Input: part model. Units: mm. Frame: model coordinates. A direction names the side the tool comes from. Round coordinates to 2 decimals unless told otherwise and drop trailing zeros. Loops run counter-clockwise (first coordinate to the right, second up) from the corner with the lowest first, then second, coordinate; pieces in that order, holes last. Notation, with made-up numbers: (-21.75, 20.25) -> (-12.75, 20.25) arc R22 ccw to (-12.75, 59.25) -> close; hole circle Ø5 at (19, 33.5). An arc over 180 degrees is marked (long way). One line per question, with ' | ' between items. Start each with the question number.
Q1. Cut plane B-B on z = -56. State how many separate pieces and enclosed holes the cut face has, and give its area (3 significant figures).
Q2. Access query for faces 1 (the face through (338, -104, 10)), 2 (the face through (310, -101, -1)), 3 (the face through (10, -94, 59)). Directions: +Z, -Z, +X, -X, +Y, -Y. A direction counts if a zero-diameter tool reaches every point of the face in a straight line with its end or side. Return the directions, or none.
Q3. Cut plane A-A on x = 233.5. Return loops of the section in (y, z).
Q4. Material intervals for L1, parallel to Y at x = 18.5, z = 80.5; L2, parallel to X at y = -103.5, z = 90; L3, parallel to X at y = 5, z = -18, sorted ascending.
Q5. Mould query, pull axis X, two halves, no side actions, for faces 4 (the face through (307.15, -101.4, 101.99)), 5 (the face through (205, 114, 116)). Classes: pulls with the +X half, pulls with the -X half, needs draft (parallel to the pull), parting line crosses it, or undercut.
Q6. Contact query for flat-ended pins moving along their axis: P1, Ø4, axis at y = -29, z = 47.5, coming from the -X side; P2, Ø8, axis at x = 191, y = -87.5, coming from the +Z side; P3, Ø10, axis at y = -101.5, z = 44, coming from the -X side; P4, Ø4, axis at x = 328, z = -9.5, coming from the +Y side. Output: stop coordinate, or through.
Q7. Cut plane D-D on y = 65.5. Return loops of the section in (x, z), and give its area (3 significant figures).
Q8. Cut plane C-C on x = 38. Return loops of the section in (y, z).
from build123d import *

# Parameters (mm, degrees)
SKETCH1_W            = 20
SKETCH1_H            = 260
BOSS_EXTRUDE1_DEPTH  = 10
CUT_EXTRUDE1_DEPTH   = 15
SKETCH3_W            = 10
SKETCH3_H            = 20
BOSS_EXTRUDE2_DEPTH  = 40
BOSS_EXTRUDE3_DEPTH  = 230
BOSS_EXTRUDE4_DEPTH  = 50
SKETCH6_W            = 260
SKETCH6_H            = 228
BOSS_EXTRUDE5_DEPTH  = 20
SKETCH7_W            = 20
SKETCH7_H            = 17
BOSS_EXTRUDE6_DEPTH  = 50
SKETCH8_W            = 20
SKETCH8_H            = 60
BOSS_EXTRUDE7_DEPTH  = 50
SKETCH9_W            = 20
SKETCH9_H            = 60
BOSS_EXTRUDE8_DEPTH  = 50
SKETCH10_W           = 20
SKETCH10_H           = 20
BOSS_EXTRUDE9_DEPTH  = 340
SKETCH11_W           = 20
SKETCH11_H           = 20
BOSS_EXTRUDE10_DEPTH = 340
SKETCH12_W           = 260
SKETCH12_H           = 228
BOSS_EXTRUDE11_DEPTH = 20
SKETCH13_W           = 40
SKETCH13_H           = 20
CUT_EXTRUDE2_DEPTH   = 240
SKETCH14_W           = 210
SKETCH14_H           = 15
CUT_EXTRUDE3_DEPTH   = 230
SKETCH15_W           = 100
SKETCH15_H           = 20
CUT_EXTRUDE4_DEPTH   = 45
SKETCH16_W           = 20
SKETCH16_H           = 100
CUT_EXTRUDE5_DEPTH   = 84
SKETCH17_W           = 20
SKETCH17_H           = 100
CUT_EXTRUDE6_DEPTH   = 84
SKETCH18_W           = 20
SKETCH18_H           = 84
CUT_EXTRUDE7_DEPTH   = 100
SKETCH19_W           = 100
SKETCH19_H           = 20
CUT_EXTRUDE8_DEPTH   = 45
CUT_EXTRUDE9_REACH   = 475.244
SKETCH20_W           = 50
SKETCH20_H           = 40
SKETCH21_W           = 50
SKETCH21_H           = 40
CUT_EXTRUDE10_DEPTH  = 18
CUT_EXTRUDE11_REACH  = 475.244
SKETCH22_W           = 50
SKETCH22_H           = 40
SKETCH23_W           = 50
SKETCH23_H           = 40
CUT_EXTRUDE12_DEPTH  = 18
CUT_EXTRUDE13_DEPTH  = 400.369503092
CUT_EXTRUDE14_DEPTH  = 400.369503092
CUT_EXTRUDE15_REACH  = 419.488
FILLET1_R            = 10


with BuildPart() as part:
    # Sketch1 → Boss-Extrude1 (new body)
    with BuildSketch(Plane(origin=(70, 0, 0), x_dir=(0, -1, 0), z_dir=(-1, 0, 0))):
        with Locations((104, 0)):
            Rectangle(SKETCH1_W, SKETCH1_H)
    extrude(amount=-BOSS_EXTRUDE1_DEPTH)

    # Sketch2 → Cut-Extrude1 (cut)
    with BuildSketch(Plane(origin=(0, -94, 0), x_dir=(-1, 0, 0), z_dir=(0, 1, 0))):
        with BuildLine():
            Line((-80, 105), (-80, -105))
            ThreePointArc((-80, -105), (-72.928932188, -102.071067812), (-70, -95))
            Line((-70, -95), (-70, 95))
            ThreePointArc((-70, 95), (-72.928932188, 102.071067812), (-80, 105))
        make_face()
    extrude(amount=-CUT_EXTRUDE1_DEPTH, mode=Mode.SUBTRACT)

    # Sketch3 → Boss-Extrude2 (add)
    with BuildSketch(Plane(origin=(0, -94, 0), x_dir=(-1, 0, 0), z_dir=(0, 1, 0))):
        with Locations((-75, -120)):
            Rectangle(SKETCH3_W, SKETCH3_H)
    extrude(amount=BOSS_EXTRUDE2_DEPTH)

    # Sketch4 → Boss-Extrude3 (add)
    with BuildSketch(Plane(origin=(80, 0, 0), x_dir=(0, 0, -1), z_dir=(1, 0, 0))):
        Polygon((-130, -114), (-130, -94), (110, -94), (110, -54), (130, -54), (130, -114), align=None)
    extrude(amount=BOSS_EXTRUDE3_DEPTH)

    # Sketch5 → Boss-Extrude4 (add)
    with BuildSketch(Plane(origin=(310, 0, 0), x_dir=(0, 0, -1), z_dir=(1, 0, 0))):
        Polygon((110, -94), (110, -54), (130, -54), (130, -114), (-130, -114), (-130, -54), (-110, -54), (-110, -94), align=None)
    extrude(amount=BOSS_EXTRUDE4_DEPTH)

    # Sketch6 → Boss-Extrude5 (add)
    with BuildSketch(Plane(origin=(360, 0, 0), x_dir=(0, 0, -1), z_dir=(1, 0, 0))):
        Rectangle(SKETCH6_W, SKETCH6_H)
        Polygon((92.025912459, -94), (0, -13.30035369), (-92.025912459, -94), align=None, mode=Mode.SUBTRACT)
    extrude(amount=BOSS_EXTRUDE5_DEPTH)

    # Sketch7 → Boss-Extrude6 (add)
    with BuildSketch(Plane.ZY.offset(-70)):
        with Locations((0, -105.5)):
            Rectangle(SKETCH7_W, SKETCH7_H)
    extrude(amount=BOSS_EXTRUDE6_DEPTH)

    # Sketch8 → Boss-Extrude7 (add)
    with BuildSketch(Plane.ZY.offset(-70)):
        with Locations((120, -84)):
            Rectangle(SKETCH8_W, SKETCH8_H)
    extrude(amount=BOSS_EXTRUDE7_DEPTH)

    # Sketch9 → Boss-Extrude8 (add)
    with BuildSketch(Plane.ZY.offset(-70)):
        with Locations((-120, -84)):
            Rectangle(SKETCH9_W, SKETCH9_H)
    extrude(amount=BOSS_EXTRUDE8_DEPTH)

    # Sketch10 → Boss-Extrude9 (add)
    with BuildSketch(Plane.ZY.offset(-360)):
        with Locations((-120, 104)):
            Rectangle(SKETCH10_W, SKETCH10_H)
    extrude(amount=BOSS_EXTRUDE9_DEPTH)

    # Sketch11 → Boss-Extrude10 (add)
    with BuildSketch(Plane.ZY.offset(-360)):
        with Locations((120, 104)):
            Rectangle(SKETCH11_W, SKETCH11_H)
    extrude(amount=BOSS_EXTRUDE10_DEPTH)

    # Sketch12 → Boss-Extrude11 (add)
    with BuildSketch(Plane(origin=(20, 0, 0), x_dir=(0, 0, -1), z_dir=(1, 0, 0))):
        Rectangle(SKETCH12_W, SKETCH12_H)
        Polygon((10, 8.769230769), (10, 10), (11.403508772, 10), align=None, mode=Mode.SUBTRACT)
        Polygon((-10, -94), (-110, -94), (-110, -10), (-11.403508772, -10), (-10, -8.769230769), align=None, mode=Mode.SUBTRACT)
    extrude(amount=-BOSS_EXTRUDE11_DEPTH)

    # Sketch13 → Cut-Extrude2 (cut)
    with BuildSketch(Plane(origin=(70, 0, 0), x_dir=(0, -1, 0), z_dir=(-1, 0, 0))):
        with Locations((74, -120)):
            Rectangle(SKETCH13_W, SKETCH13_H)
    extrude(amount=-CUT_EXTRUDE2_DEPTH, mode=Mode.SUBTRACT)

    # Sketch14 → Cut-Extrude3 (cut)
    with BuildSketch(Plane.ZY.offset(-80)):
        with Locations((0, -101.5)):
            Rectangle(SKETCH14_W, SKETCH14_H)
    extrude(amount=-CUT_EXTRUDE3_DEPTH, mode=Mode.SUBTRACT)

    # Sketch15 → Cut-Extrude4 (cut)
    with BuildSketch(Plane(origin=(360, 0, 0), x_dir=(0, 0, -1), z_dir=(1, 0, 0))):
        with Locations((60, -104)):
            Rectangle(SKETCH15_W, SKETCH15_H)
    extrude(amount=-CUT_EXTRUDE4_DEPTH, mode=Mode.SUBTRACT)

    # Sketch16 → Cut-Extrude5 (cut)
    with BuildSketch(Plane.XZ.offset(-10)):
        with Locations((10, 60)):
            Rectangle(SKETCH16_W, SKETCH16_H)
    extrude(amount=-CUT_EXTRUDE5_DEPTH, mode=Mode.SUBTRACT)

    # Sketch17 → Cut-Extrude6 (cut)
    with BuildSketch(Plane.XZ.offset(-10)):
        with Locations((10, -60)):
            Rectangle(SKETCH17_W, SKETCH17_H)
    extrude(amount=-CUT_EXTRUDE6_DEPTH, mode=Mode.SUBTRACT)

    # Sketch18 → Cut-Extrude7 (cut)
    with BuildSketch(Plane(origin=(0, 0, -110), x_dir=(-1, 0, 0), z_dir=(0, 0, -1))):
        with Locations((-10, -52)):
            Rectangle(SKETCH18_W, SKETCH18_H)
    extrude(amount=-CUT_EXTRUDE7_DEPTH, mode=Mode.SUBTRACT)

    # Sketch19 → Cut-Extrude8 (cut)
    with BuildSketch(Plane(origin=(360, 0, 0), x_dir=(0, 0, -1), z_dir=(1, 0, 0))):
        with Locations((-60, -104)):
            Rectangle(SKETCH19_W, SKETCH19_H)
    extrude(amount=-CUT_EXTRUDE8_DEPTH, mode=Mode.SUBTRACT)

    # Sketch20 → Cut-Extrude9 (cut, up to next)
    with BuildSketch(Plane(origin=(0, 0, -128), x_dir=(-1, 0, 0), z_dir=(0, 0, -1)), mode=Mode.PRIVATE) as cut_extrude9_sk1:
        with Locations((-45, -74)):
            Rectangle(SKETCH20_W, SKETCH20_H)
    cut_extrude9_tool1 = extrude(cut_extrude9_sk1.sketch, amount=-CUT_EXTRUDE9_REACH, mode=Mode.PRIVATE) & part.part
    add(cut_extrude9_tool1.solids().sort_by_distance((45, -74, -128))[0], mode=Mode.SUBTRACT)

    # Sketch21 → Cut-Extrude10 (cut)
    with BuildSketch(Plane.XY.offset(-110)):
        with Locations((335, -74)):
            Rectangle(SKETCH21_W, SKETCH21_H)
    extrude(amount=-CUT_EXTRUDE10_DEPTH, mode=Mode.SUBTRACT)

    # Sketch22 → Cut-Extrude11 (cut, up to next)
    with BuildSketch(Plane.XY.offset(128), mode=Mode.PRIVATE) as cut_extrude11_sk1:
        with Locations((45, -74)):
            Rectangle(SKETCH22_W, SKETCH22_H)
    cut_extrude11_tool1 = extrude(cut_extrude11_sk1.sketch, amount=-CUT_EXTRUDE11_REACH, mode=Mode.PRIVATE) & part.part
    add(cut_extrude11_tool1.solids().sort_by_distance((45, -74, 128))[0], mode=Mode.SUBTRACT)

    # Sketch23 → Cut-Extrude12 (cut)
    with BuildSketch(Plane(origin=(0, 0, 110), x_dir=(-1, 0, 0), z_dir=(0, 0, -1))):
        with Locations((-335, -74)):
            Rectangle(SKETCH23_W, SKETCH23_H)
    extrude(amount=-CUT_EXTRUDE12_DEPTH, mode=Mode.SUBTRACT)

    # Sketch24 → Cut-Extrude13 (cut, through all)
    with BuildSketch(Plane.ZY.offset(-360)):
        Polygon((-92.025912459, 94), (0, 13.30035369), (92.025912459, 94), align=None)
    extrude(amount=-CUT_EXTRUDE13_DEPTH, mode=Mode.SUBTRACT)

    # Sketch25 → Cut-Extrude14 (cut, through all)
    with BuildSketch(Plane.ZY.offset(-360)):
        Polygon((110, 83.161184771), (15.167069998, 0), (110, -83.161184771), align=None)
    extrude(amount=-CUT_EXTRUDE14_DEPTH, mode=Mode.SUBTRACT)

    # Sketch26 → Cut-Extrude15 (cut, up to next)
    with BuildSketch(Plane(origin=(380, 0, 0), x_dir=(0, 0, -1), z_dir=(1, 0, 0)), mode=Mode.PRIVATE) as cut_extrude15_sk1:
        Polygon((15.167069998, 0), (110, -83.161184771), (110, 83.161184771), align=None)
    cut_extrude15_tool1 = extrude(cut_extrude15_sk1.sketch, amount=-CUT_EXTRUDE15_REACH, mode=Mode.PRIVATE) & part.part
    add(cut_extrude15_tool1.solids().sort_by_distance((380, 0, -78.389023))[0], mode=Mode.SUBTRACT)

    # Fillet1
    fillet1_edges = [part.edges().sort_by_distance(p)[0] for p in [
        (310, -101.5, -105),
        (310, -101.5, 105),
    ]]
    fillet(fillet1_edges, radius=FILLET1_R)


solid = part.part
Results:
1) separate pieces: 8 | enclosed holes: 0 | area: 4,360 mm^2
2) face 1: +Y, -Y | face 2: +Y | face 3: -X
3) outline: (-114, -130) -> (-94, -130) -> (-94, -105) -> (-109, -105) -> (-109, 105) -> (-94, 105) -> (-94, 130) -> (-114, 130) -> close; (94, -130) -> (114, -130) -> (114, -110) -> (94, -110) -> close; (94, 110) -> (114, 110) -> (114, 130) -> (94, 130) -> close
4) L1: -114 to -94, -10 to 10, 94 to 114 | L2: 0 to 20, 310 to 315, 360 to 380 | L3: 0 to 20, 360 to 380
5) face 4: undercut | face 5: needs draft
6) P1: x = 360 | P2: through | P3: x = 0 | P4: y = -94
7) outline: (0, -130) -> (20, -130) -> (20, -110) -> (0, -110) -> close; (0, -10) -> (20, -10) -> (20, 10) -> (0, 10) -> close; (0, 110) -> (20, 110) -> (20, 130) -> (0, 130) -> close; (360, -130) -> (380, -130) -> (380, -110) -> (360, -110) -> close; (360, -89.86) -> (380, -89.86) -> (380, -59.53) -> (360, -59.53) -> close; (360, 59.53) -> (380, 59.53) -> (380, 89.86) -> (360, 89.86) -> close; (360, 110) -> (380, 110) -> (380, 130) -> (360, 130) -> close | area: 3,210 mm^2
8) outline: (-114, -130) -> (-54, -130) -> (-54, -128) -> (-94, -128) -> (-94, -110) -> (-114, -110) -> close; (-114, -10) -> (-97, -10) -> (-97, 10) -> (-114, 10) -> close; (-114, 110) -> (-94, 110) -> (-94, 128) -> (-54, 128) -> (-54, 130) -> (-114, 130) -> close; (94, -130) -> (114, -130) -> (114, -110) -> (94, -110) -> close; (94, 110) -> (114, 110) -> (114, 130) -> (94, 130) -> close
